Job drawing, mm, ordinate dimensions from the low corner. One solid piece. A direction names the side the tool comes from. Give positions to 0.01 mm unless a question says otherwise; leave off trailing zeros. Order: outer loops, then holes, each group sorted by start corner. A loop starts at its lowest first (then second) coordinate and runs counter-clockwise, first axis right, second up. Notation, with made-up numbers: (-7, 64.25) - (-1, 64.25) arc R23 ccw to (-1, 100.25) - close; hole circle Ø3 at (84.25, 84.5). An arc over 180 degrees is marked (long way). Write each question's results on one line, items separated by ' | '. Start each with the question number.
1) Two-plate mould, pull along X, no slides. Class the marked faces 1, 2 and 3: +X half, -X half, draft (parallel to the pull), parting line (faces both ways), or undercut.
2) Cut at A-A on x = 12.5. List the corners of the cut face in (y, z).
3) Drop flat-ended pins along their axis: pin 1 Ø6 at (y, z) = (13, 18.5) entering from -X; pin 2 Ø5 at (x, y) = (10, 7.5) entering from +Z; pin 3 Ø6 at (x, z) = (13.5, 5.5) entering from -Y; pin 4 Ø7 at (x, z) = (17, 8.5) entering from +Y. Give the stop position or say it passes through.
4) Cut at C-C on y = 4.5. List the corners of the cut face in (x, z).
5) Drill centre lines: line 1 along Y through (x, z) = (21.5, 0.45); line 2 along X through (y, z) = (20, 2.5); line 3 along Z through (x, y) = (12.5, 0.5). Where is each one in solid material? Low to high. Write a range as from..to.
6) Cut at D-D on z = 16.5. List the corners of the cut face in (x, y).
7) Tool access for the marked faces 4 and 5: list every direction of +Z, -Z, +X, -X, +Y, -Y with a clear straight run to the whole face (end or side of a thin tool).
8) Cut at B-B on x = 3.5. List the corners of the cut face in (y, z), plus the area to 3 significant figures.
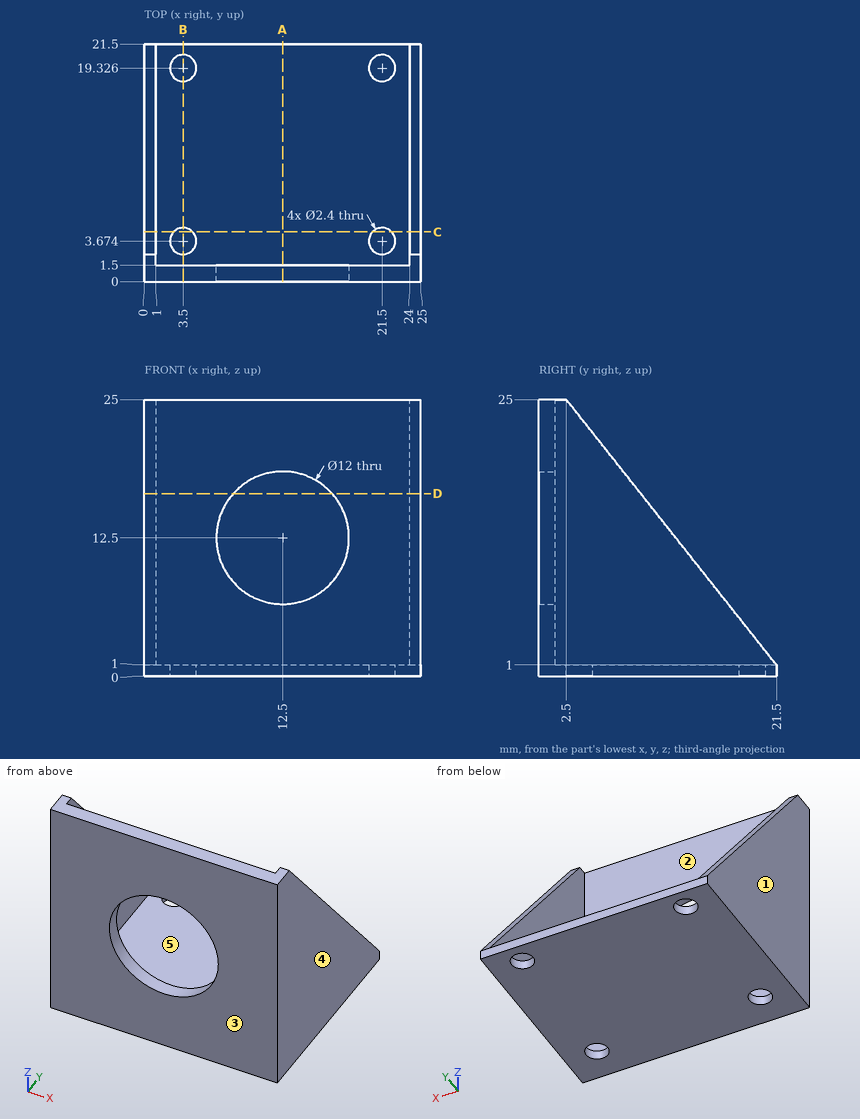
Results:
1) face 1: -X half | face 2: undercut | face 3: draft
2) outline: (0, 0) - (21.5, 0) - (21.5, 1) - (1.5, 1) - (1.5, 6.5) - (0, 6.5) - close; (0, 18.5) - (1.5, 18.5) - (1.5, 25) - (0, 25) - close
3) pin 1: through | pin 2: z = 1 | pin 3: y = 0 | pin 4: y = 1.5
4) outline: (0, 0) - (2.63, 0) - (2.63, 1) - (1, 1) - (1, 22.47) - (0, 22.47) - close; (4.37, 0) - (20.63, 0) - (20.63, 1) - (4.37, 1) - close; (22.37, 0) - (25, 0) - (25, 22.47) - (24, 22.47) - (24, 1) - (22.37, 1) - close
5) line 1: 0..2.47, 4.87..18.13, 20.53..21.5 | line 2: 0..1, 24..25 | line 3: 0..6.5, 18.5..25
6) outline: (0, 0) - (8.03, 0) - (8.03, 1.5) - (1, 1.5) - (1, 9.23) - (0, 9.23) - close; (16.97, 0) - (25, 0) - (25, 9.23) - (24, 9.23) - (24, 1.5) - (16.97, 1.5) - close
7) face 4: +Z, -Z, +X, +Y, -Y | face 5: +Z, +Y
8) outline: (0, 0) - (2.47, 0) - (2.47, 1) - (1.5, 1) - (1.5, 25) - (0, 25) - close; (4.87, 0) - (18.13, 0) - (18.13, 1) - (4.87, 1) - close; (20.53, 0) - (21.5, 0) - (21.5, 1) - (20.53, 1) - close | area: 52.7 mm^2
